from build123d import *

# Parameters (mm, degrees)
ESQUISSE1_R      = 2
ESQUISSE1_R_2    = 11
EXTRUSION1_DEPTH = 3


with BuildPart() as part:
    # Esquisse1 → Extrusion1 (new body)
    with BuildSketch(Plane(origin=(0, 0, 0), x_dir=(1, 0, 0), z_dir=(0, 1, 0))):
        with BuildLine():
            Line((80.5, 0), (-80.5, 0))
            Line((-80.5, 0), (-80.5, 83))
            Line((-80.5, 83), (-115.5, 83))
            Line((-115.5, 83), (-115.5, 96))
            Line((-115.5, 96), (-125.5, 96))
            Line((-125.5, 96), (-125.5, 206))
            Line((-125.5, 206), (-93.5, 206))
            ThreePointArc((-93.5, 206), (0, 112.5), (93.5, 206))
            Line((93.5, 206), (125.5, 206))
            Line((125.5, 206), (125.5, 96))
            Line((125.5, 96), (115.5, 96))
            Line((115.5, 96), (115.5, 83))
            Line((115.5, 83), (80.5, 83))
            Line((80.5, 83), (80.5, 0))
        make_face()
        with Locations((94.89, 146.61)):
            Circle(ESQUISSE1_R, mode=Mode.SUBTRACT)
        with Locations((-105.5, 136)):
            Circle(ESQUISSE1_R_2, mode=Mode.SUBTRACT)
        with Locations((-116.11, 146.61)):
            Circle(ESQUISSE1_R, mode=Mode.SUBTRACT)
        with Locations((-116.11, 125.39)):
            Circle(ESQUISSE1_R, mode=Mode.SUBTRACT)
        with Locations((-94.89, 125.39)):
            Circle(ESQUISSE1_R, mode=Mode.SUBTRACT)
        with Locations((-94.89, 146.61)):
            Circle(ESQUISSE1_R, mode=Mode.SUBTRACT)
        with Locations((94.89, 125.39)):
            Circle(ESQUISSE1_R, mode=Mode.SUBTRACT)
        with Locations((116.11, 125.39)):
            Circle(ESQUISSE1_R, mode=Mode.SUBTRACT)
        with Locations((116.11, 146.61)):
            Circle(ESQUISSE1_R, mode=Mode.SUBTRACT)
        with Locations((105.5, 136)):
            Circle(ESQUISSE1_R_2, mode=Mode.SUBTRACT)
    extrude(amount=EXTRUSION1_DEPTH)


solid = part.part
Can you work these out from the model? Positions are in its coordinate system, mm. Coordinates: 2 decimals unless noted, no trailing zeros. Order: outer loops, then holes, each group sorted by start corner. A loop starts at its lowest first (then second) coordinate and runs counter-clockwise, first axis right, second up. Notation, with made-up numbers: M -30,17.25 L -11,17.25 A11 ccw -11,37.25 Z; hole C 52,-35 d5. An arc over 180 degrees is marked long. Answer as CSV lines item,"result".
(1) Suppose I cut it at D-D on z = -173. Please give me the cut outline in (x, y).
Geometry check:
outline,"M -125.5,0 L -87.48,0 L -87.48,3 L -125.5,3 Z; M 87.48,0 L 125.5,0 L 125.5,3 L 87.48,3 Z"
(2) I'm going to push flat-ended pins straight in: pin 1 (0.9 mm diameter, centred on y = 1.5, z = -89, fed in from -X); pin 2 (3 mm diameter, centred on x = -116.11, z = -146.61, fed in from +Y); pin 3 (0.9 mm diameter, centred on x = 102.5, y = 1, fed in from +Z); pin 4 (1.5 mm diameter, centred on y = 2, z = -45.5, fed in from +X). Where does each tip first touch, or does it pass through?
Geometry check:
pin 1,"x = -115.5"
pin 2,"through"
pin 3,"z = -83"
pin 4,"x = 80.5"
(3) Please list where these lines run through material, in increasing order: L1, parallel to X at y = 1.25, z = -136; L2, parallel to Z at x = 105.5, y = 1.1; L3, parallel to X at y = 0.9, z = -34.5.
Geometry check:
L1,"-125.5 to -116.5, -94.5 to -61.99, 61.99 to 94.5, 116.5 to 125.5"
L2,"-206 to -147, -125 to -83"
L3,"-80.5 to 80.5"
(4) Suppose I cut it at A-A on x = -105.5. Please give me the cut outline in (y, z).
Geometry check:
outline,"M 0,-206 L 3,-206 L 3,-147 L 0,-147 Z; M 0,-125 L 3,-125 L 3,-83 L 0,-83 Z"
(5) Suppose I cut it at B-B on y = 1.85. Count the separate pieces of the cut face and the enclosed holes in it, plus the area to 3 significant figures.
Geometry check:
separate pieces,"1"
enclosed holes,"10"
area,"29,400 mm^2"
(6) Suppose I cut it at C-C on z = -136. Please give me the cut outline in (x, y).
Geometry check:
outline,"M -125.5,0 L -116.5,0 L -116.5,3 L -125.5,3 Z; M -94.5,0 L -61.99,0 L -61.99,3 L -94.5,3 Z; M 61.99,0 L 94.5,0 L 94.5,3 L 61.99,3 Z; M 116.5,0 L 125.5,0 L 125.5,3 L 116.5,3 Z"
(7) If we mould it in two halves opening along X, with no side actions, what happens to faces 1 (the cylindrical face through (-2.056, 1.479, -112.523)), 2 (the cylindrical face through (97.39, 1.48, -143.43)), 3 (the flat face through (2, 0, -82))? For each: released by +X, released by -X, zero draft, split by the parting line, or undercut.
Geometry check:
face 1,"undercut"
face 2,"undercut"
face 3,"zero draft"
